CAD build for the part. Positions are in the model's coordinates, mm. A direction names the side the tool comes from. Coordinates: 2 decimals unless noted, no trailing zeros. Loops run counter-clockwise (first coordinate to the right, second up) from the corner with the lowest first, then second, coordinate; pieces in that order, holes last. Notation, with made-up numbers: (-17.5, 40.5) -> (23.5, 40.5) arc R20 ccw to (23.5, 45.5) -> close; hole circle Ø9 at (12, 3). An arc over 180 degrees is marked (long way). Write item = value, one per line. Start each with the question number.
(1) Band-saw the part on A-A (x = -6). Write the cut outline in (y, z), and give its area (3 significant figures).
(2) Pull direction X, two halves, no side cores. Call faces 1 (the face through (-1, 120, 1)), 2 (the face through (-51.722, 120, 20)), 3 (the face through (0, 120, 5)): +X half, -X half, draft (parallel to the pull), parting line (faces both ways), or undercut.
(3) Drill centre lines: line 1 (X direction, y = 123.75, z = 31.5); line 2 (Z direction, x = -23, y = 122.5). Where is each one in solid material? Low to high. Write a range as from..to.
(4) Band-saw the part on C-C (y = 121.25). Write the cut outline in (x, z).
(5) Tool access for faces 4 (the face through (0, 120, 35)), 5 (the face through (1, 124.867, 3)): list every direction of +Z, -Z, +X, -X, +Y, -Y with a clear straight run to the whole face (end or side of a thin tool).
(6) Band-saw the part on B-B (z = 29.5). Write the cut outline in (x, y).
```python
from build123d import *

# Parameters (mm, degrees)
SKETCH5_W           = 103.443318868
SKETCH5_H           = 10
EXTRUDE_THIN1_DEPTH = 66
SKETCH7_W           = 67.24350567
SKETCH7_H           = 56
CUT_EXTRUDE2_DEPTH  = 10
SKETCH8_W           = 67.24350567
SKETCH8_H           = 10
BOSS_EXTRUDE1_DEPTH = 26
SKETCH9_W           = 103.443318868
SKETCH9_H           = 27
SKETCH9_H_2         = 1
CUT_EXTRUDE3_DEPTH  = 10


with BuildPart() as part:
    # Sketch5 → Extrude-Thin1 (new body)
    with BuildSketch(Plane.XY):
        with Locations((0, 119.867131674)):
            Rectangle(SKETCH5_W, SKETCH5_H)
    extrude(amount=EXTRUDE_THIN1_DEPTH)

    # Sketch7 → Cut-Extrude2 (cut)
    with BuildSketch(Plane(origin=(0, 124.867131674, 0), x_dir=(1, 0, 0), z_dir=(0, 1, 0))):
        with Locations((0, -33)):
            Rectangle(SKETCH7_W, SKETCH7_H)
    extrude(amount=-CUT_EXTRUDE2_DEPTH, mode=Mode.SUBTRACT)

    # Sketch8 → Boss-Extrude1 (add)
    with BuildSketch(Plane(origin=(0, 0, 61), x_dir=(-1, 0, 0), z_dir=(0, 0, -1))):
        with Locations((0, 119.867131674)):
            Rectangle(SKETCH8_W, SKETCH8_H)
    extrude(amount=BOSS_EXTRUDE1_DEPTH)

    # Sketch9 → Cut-Extrude3 (cut)
    with BuildSketch(Plane(origin=(0, 124.867131674, 0), x_dir=(1, 0, 0), z_dir=(0, 1, 0))):
        with Locations((0, -52.5)):
            Rectangle(SKETCH9_W, SKETCH9_H)
        with Locations((0, -0.5)):
            Rectangle(SKETCH9_W, SKETCH9_H_2)
    extrude(amount=-CUT_EXTRUDE3_DEPTH, mode=Mode.SUBTRACT)


solid = part.part
```
Findings below:
q1.outline = (114.87, 1) -> (124.87, 1) -> (124.87, 5) -> (114.87, 5) -> close; (114.87, 35) -> (124.87, 35) -> (124.87, 39) -> (114.87, 39) -> close
q1.area = 80.0 mm²
q2.face_1 = draft
q2.face_2 = -X half
q2.face_3 = undercut
q3.line_1 = -51.72..-33.62, 33.62..51.72
q3.line_2 = 1..5, 35..39
q4.outline = (-51.72, 1) -> (51.72, 1) -> (51.72, 39) -> (-51.72, 39) -> close; hole (-33.62, 5) -> (33.62, 5) -> (33.62, 35) -> (-33.62, 35) -> close
q5.face_4 = +Y, -Y
q5.face_5 = +Z, -Z, +X, -X, +Y
q6.outline = (-51.72, 114.87) -> (-33.62, 114.87) -> (-33.62, 124.87) -> (-51.72, 124.87) -> close; (33.62, 114.87) -> (51.72, 114.87) -> (51.72, 124.87) -> (33.62, 124.87) -> close
